Design review of the part built by this model. Coordinates are the model's own, in mm. A direction names the side the tool comes from. Coordinates: 2 decimals unless noted, no trailing zeros. Loops run counter-clockwise (first coordinate to the right, second up) from the corner with the lowest first, then second, coordinate; pieces in that order, holes last. Notation, with made-up numbers: M 29.5,-1.75 L 77.5,-1.75 A28 ccw 77.5,17.25 Z; hole C 82.5,25.25 d9. An arc over 180 degrees is marked long. Answer as a JSON object with one key per item and string values. Group by question number.
1. Consider section D-D (x = 6). State the section outline as (y, z) points.
2. Insertion check: pin 1 (8 mm diameter, centred on x = 8, z = 22, fed in from +Y); pin 2 (3.5 mm diameter, centred on y = 33, z = 13.5, fed in from -X); pin 3 (21 mm diameter, centred on x = -6, z = 29.5, fed in from -Y); pin 4 (8 mm diameter, centred on x = 3.5, y = -18, fed in from +Z). Each pin has a flat end and moves straight along its axis. Give the tip position at first contact, or say it passes through.
3. Consider section B-B (y = -14.5). State the section outline as (x, z) points.
4. Draft analysis for pull direction Y (two halves, no side actions). For faces 6 (the flat face through (-1, 1, 40)), 7 (the flat face through (-9, -6, 20)), 8 (the cylindrical face through (9.498, 14.313, 20.28)), 9 (the flat face through (-8, 28, 20)), state which applies: +Y half, -Y half, draft (parallel to the pull), parting line (faces both ways), or undercut.
5. Machinability: for faces 1 (the flat face through (21.5, 34, 20)), 2 (the cylindrical face through (9.498, -14.313, 20.28)), 3 (the flat face through (29, 40, 20)), 4 (the flat face through (29, -40, 20)), 5 (the flat face through (21.5, -34, 20)), which of the approach directions +Z, -Z, +X, -X, +Y, -Y give a long, thin tool a straight path to every point of the face, cutting with its end or side? Answer none if there is none.
6. Consider section A-A (z = 7.5). State the section outline as (x, y) points.
7. To check wall thickness, follow probe 1 along Y at (x, z) = (-12, 2.5); probe 2 along Y at (x, z) = (-23.5, 3); probe 3 along X at (y, z) = (17, 9). State the ranges of each line that lie inside material, in increasing order.
8. Consider section C-C (x = 17.5). State the section outline as (y, z) points.
from build123d import *

# Parameters (mm, degrees)
SKETCH_1_W          = 73
SKETCH_1_H          = 80
EXTRUDE_1_DEPTH     = 40
SKETCH_2_R          = 21.5
CUT_EXTRUDE_1_DEPTH = 68.321987493
SKETCH_3_W          = 58
SKETCH_3_H          = 12
CUT_EXTRUDE_5_DEPTH = 68.321987493


with BuildPart() as part:
    # Эскиз1 → Бобышка-Вытянуть1 (new body)
    with BuildSketch(Plane.XY):
        Rectangle(SKETCH_1_W, SKETCH_1_H)
    extrude(amount=EXTRUDE_1_DEPTH)

    # Эскиз2 → Вырез-Вытянуть1 (cut, through all)
    with BuildSketch(Plane.XY.offset(40)):
        with Locations((36.5, 0)):
            Circle(SKETCH_2_R)
        with BuildLine():
            Line((-18, -6), (1, -6))
            ThreePointArc((1, -6), (9.5, -14.5), (1, -23))
            Line((1, -23), (-18, -23))
            ThreePointArc((-18, -23), (-26.5, -14.5), (-18, -6))
        make_face()
        with BuildLine():
            Line((-18, 6), (1, 6))
            ThreePointArc((1, 6), (9.5, 14.5), (1, 23))
            Line((1, 23), (-18, 23))
            ThreePointArc((-18, 23), (-26.5, 14.5), (-18, 6))
        make_face()
    extrude(amount=-CUT_EXTRUDE_1_DEPTH, mode=Mode.SUBTRACT)

    # Эскиз3 → Вырез-Вытянуть5 (cut, through all)
    with BuildSketch(Plane.XY.offset(40)):
        with Locations((-7.5, 34)):
            Rectangle(SKETCH_3_W, SKETCH_3_H)
    cut_extrude_5 = extrude(amount=-CUT_EXTRUDE_5_DEPTH, mode=Mode.SUBTRACT)

    # Зеркальное отражение1: Вырез-Вытянуть5 across plane
    add(cut_extrude_5.mirror(Plane.ZX), mode=Mode.SUBTRACT)


solid = part.part
Findings below:
{
 "1": {"outline": "M -28,0 L -21.37,0 L -21.37,40 L -28,40 Z; M -7.63,0 L 7.63,0 L 7.63,40 L -7.63,40 Z; M 21.37,0 L 28,0 L 28,40 L 21.37,40 Z"},
 "2": {"pin 1": "stops at y = 28", "pin 2": "stops at x = 21.5", "pin 3": "stops at y = -28", "pin 4": "passes through"},
 "3": {"outline": "M -36.5,0 L -26.5,0 L -26.5,40 L -36.5,40 Z; M 9.5,0 L 20.63,0 L 20.63,40 L 9.5,40 Z"},
 "4": {"face 6": "draft", "face 7": "undercut", "face 8": "undercut", "face 9": "+Y half"},
 "5": {"face 1": "+Z, -Z, -X, +Y", "face 2": "+Z, -Z", "face 3": "+Z, -Z, +X, -X, +Y", "face 4": "+Z, -Z, +X, -X, -Y", "face 5": "+Z, -Z, -X, -Y"},
 "6": {"outline": "M -36.5,-28 L 21.5,-28 L 21.5,-40 L 36.5,-40 L 36.5,-21.5 A21.5 cw 36.5,21.5 L 36.5,40 L 21.5,40 L 21.5,28 L -36.5,28 Z; hole M -18,-23 L 1,-23 A8.5 ccw 1,-6 L -18,-6 A8.5 ccw Z; hole M -18,6 L 1,6 A8.5 ccw 1,23 L -18,23 A8.5 ccw Z"},
 "7": {"probe 1": "y = -28 to -23, -6 to 6, 23 to 28", "probe 2": "y = -28 to -20.98, -8.02 to 8.02, 20.98 to 28", "probe 3": "x = -36.5 to -26.12, 9.12 to 23.34"},
 "8": {"outline": "M -28,0 L -10.06,0 L -10.06,40 L -28,40 Z; M 10.06,0 L 28,0 L 28,40 L 10.06,40 Z"}
}
